The model under review builds one solid part; all positions refer to its coordinate system, in mm. Coordinates: 2 decimals unless noted, no trailing zeros. Write each loop counter-clockwise with the first axis right and the second up, starting at its lowest first coordinate (ties: lowest second). Pieces come first, ordered by that corner, then holes. Notation, with made-up numbers: M -21,-19 L 0,-19 A14 ccw 0,-9 Z; hole C -10,17.25 d8. An arc over 180 degrees is marked long. Answer as a JSON object with one key per item and string values.
```python
from build123d import *

# Parameters (mm, degrees)
SKETCH_1_W          = 160
SKETCH_1_H          = 160
EXTRUDE_1_DEPTH     = 4
EXTRUDE_2_DEPTH     = 4
SKETCH_3_R          = 31
SKETCH_3_R_2        = 1.6
CUT_EXTRUDE_2_DEPTH = 10


with BuildPart() as part:
    # 草图1 → 凸台-拉伸1 (new body)
    with BuildSketch(Plane(origin=(0, 0, 0), x_dir=(1, 0, 0), z_dir=(0, 1, 0))):
        with Locations((80, 80)):
            Rectangle(SKETCH_1_W, SKETCH_1_H)
    extrude(amount=EXTRUDE_1_DEPTH)

    # 草图2 → 凸台-拉伸2 (add)
    with BuildSketch(Plane(origin=(0, 4, 0), x_dir=(1, 0, 0), z_dir=(0, 1, 0))):
        Polygon((0, 100), (-40, 140), (-40, 160), (0, 160), (0, 200), (20, 200), (60, 160), align=None)
        Polygon((60, 0), (0, 60), (-40, 20), (-40, 0), (0, 0), (0, -40), (20, -40), align=None)
        Polygon((160, 60), (200, 20), (200, 0), (160, 0), (160, -40), (140, -40), (100, 0), align=None)
        Polygon((100, 160), (160, 100), (200, 140), (200, 160), (160, 160), (160, 200), (140, 200), align=None)
    extrude(amount=-EXTRUDE_2_DEPTH)

    # 草图3 → 切除-拉伸2 (cut)
    with BuildSketch(Plane.XZ):
        with Locations(Location((80, -110, 0), (0, 0, 270))):
            Circle(SKETCH_3_R)
        with Locations(Location((80, -76, 0), (0, 0, 270))):
            Circle(SKETCH_3_R_2)
        with Locations(Location((104.04163056, -85.95836944, 0), (0, 0, 270))):
            Circle(SKETCH_3_R_2)
        with Locations(Location((114, -110, 0), (0, 0, 270))):
            Circle(SKETCH_3_R_2)
        with Locations(Location((104.04163056, -134.04163056, 0), (0, 0, 270))):
            Circle(SKETCH_3_R_2)
        with Locations(Location((80, -144, 0), (0, 0, 270))):
            Circle(SKETCH_3_R_2)
        with Locations(Location((55.95836944, -134.04163056, 0), (0, 0, 270))):
            Circle(SKETCH_3_R_2)
        with Locations(Location((46, -110, 0), (0, 0, 270))):
            Circle(SKETCH_3_R_2)
        with Locations(Location((55.95836944, -85.95836944, 0), (0, 0, 270))):
            Circle(SKETCH_3_R_2)
    extrude(amount=-CUT_EXTRUDE_2_DEPTH, mode=Mode.SUBTRACT)


solid = part.part
```
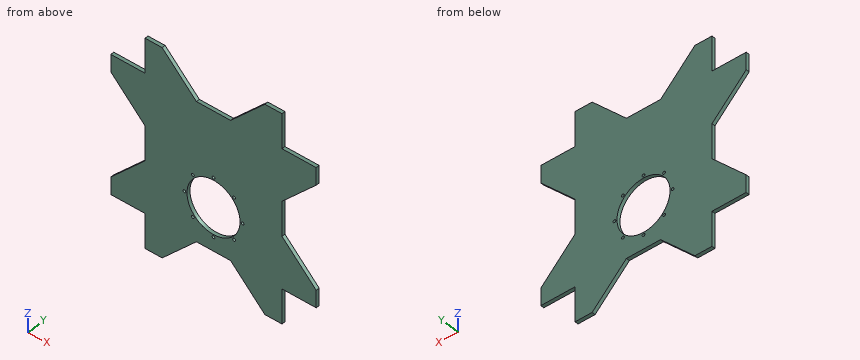
(1) For pin 1 Ø1.9 at (x, z) = (55.96, -85.96) entering from +Y; pin 2 Ø1.5 at (y, z) = (3, -85.5) entering from +X; pin 3 Ø1 at (x, y) = (104, 3) entering from -Z; pin 4 Ø2 at (y, z) = (2, -184.5) entering from -X, all flat-tipped, find the tip position at first contact; note any pin that passes through.
Results list:
{"pin 1": "through", "pin 2": "x = 160", "pin 3": "z = -164.5", "pin 4": "x = 0"}
(2) Add section A-A on z = 14.5. Give the boundary of the cut face in (x, y).
Results list:
{"outline": "M 0,0 L 45.5,0 L 45.5,4 L 0,4 Z; M 114.5,0 L 160,0 L 160,4 L 114.5,4 Z"}
(3) Add section B-B on x = 174. Give the boundary of the cut face in (y, z), and give its area (3 significant figures).
Results list:
{"outline": "M 0,-160 L 4,-160 L 4,-114 L 0,-114 Z; M 0,-46 L 4,-46 L 4,0 L 0,0 Z", "area": "368 mm²"}
(4) Add section D-D on x = 136.5. Give the boundary of the cut face in (y, z), and give its area (3 significant figures).
Results list:
{"outline": "M 0,-196.5 L 4,-196.5 L 4,36.5 L 0,36.5 Z", "area": "932 mm²"}
(5) Wall thickness on line 1 along X through (y, z) = (3.1, -110); line 2 along Z through (x, y) = (-17.5, 1.15); line 3 along X through (y, z) = (1.9, -114): over which ranges is each line inside the solid? List them lowest first. Write a range as from..to.
Results list:
{"line 1": "-10..44.4, 47.6..49, 111..112.4, 115.6..170", "line 2": "-160..-117.5, -42.5..0", "line 3": "-14..49.26, 110.74..174"}
(6) Add section C-C on z = -51.5. Give the boundary of the cut face in (x, y), and give its area (3 significant figures).
Results list:
{"outline": "M -8.5,0 L 168.5,0 L 168.5,4 L -8.5,4 Z", "area": "708 mm²"}
